Read the model definition and answer for the solid it produces. Units are mm, in the model's axes. A direction names the side the tool comes from. Give positions to 0.01 mm unless a question says otherwise; leave off trailing zeros. Order: outer loops, then holes, each group sorted by start corner. A loop starts at its lowest first (then second) coordinate and runs counter-clockwise, first axis right, second up.
Item 1: Find the intervals of material crossed by line 1 along Z through (x, y) = (12.7, 0) (3 decimals); line 2 along X through (y, z) = (-1.5, -346) (3 decimals); line 3 along Z through (x, y) = (231.5, 0) (3 decimals), in increasing order.
Item 2: A cutting plane is placed at B-B (x = 61.5). Write down the section's boundary in (y, z) (3 decimals).
Item 3: Given pin 1 Ø7.5 at (y, z) = (0, -447.675) entering from +X; pin 2 Ø1.5 at (x, y) = (140.5, 7) entering from -Z, each flat-ended and moving along its own axis, determine where each tip first touches the part or whether it passes through.
Item 4: The mould has two halves that part along X. Classify faces 1 (the face through (244.094, 0, -232)), 2 (the face through (225, 0, -457.2)), 3 (the face through (9.034, 0.133, -11.045)): +X half, -X half, draft (parallel to the pull), parting line (faces both ways), or undercut.
Item 5: A cutting plane is placed at C-C (y = 0). State how many separate pieces and enclosed holes the cut face has, plus the area to 3 significant figures.
Item 6: A cutting plane is placed at D-D (z = -101.6). Write down the section's boundary in (x, y) (3 decimals), plus the area to 3 significant figures.
Item 7: Which of the six approach directions +Z, -Z, +X, -X, +Y, -Y give full straight-line access (tool end or side, diameter ignored) to faces 4 (the face through (224.97, 1.377, -453.874)), 5 (the face through (202.556, 0.133, -212.278)), 6 (the face through (38.1, 0, -363))?
Item 8: A cutting plane is placed at A-A (z = -349). Write down the section's boundary in (x, y) (3 decimals).
from build123d import *

# Parameters (mm, degrees)
F0_W     = 168.275
F0_H     = 177.8
F1_DEPTH = 9.525
F3_D     = 12.7
F5_D     = 12.7
F7_D     = 7.9375
F8_R     = 12.7


# Not quite as in the source:
# - a length typed as a fraction of an inch, garbled in the dataset ("3 / 203.2 mm" for 3/8 in), is restored


with BuildPart() as f1:
    # F0 (on Front) → F1 (new body, symmetric)
    with BuildSketch(Plane.XZ):
        Polygon((244.094, 0), (0, 0), (0, -457.2), (38.1, -457.2), (38.1, -254), (206.375, -254), (206.375, -457.2), (244.094, -457.2), align=None)
        with Locations((122.2375, -127)):
            Rectangle(F0_W, F0_H, mode=Mode.SUBTRACT)
    extrude(amount=F1_DEPTH, both=True)

    # F3 (through all)
    with Locations(Plane.YZ.offset(244.094)):
        with Locations((0, -447.675)):
            Hole(F3_D / 2)

    # F5 (through all)
    with Locations(Plane.XZ.offset(9.525)):
        with Locations((12.7, -406.4), (12.7, -101.6)):
            Hole(F5_D / 2)

    # F7 (through all)
    with Locations(Plane.XZ.offset(9.525)):
        with Locations((12.7, -9.525), (12.7, -28.575), (231.394, -28.575), (231.394, -9.525)):
            Hole(F7_D / 2)

    # F8
    f8_edges = [f1.edges().sort_by_distance(p)[0] for p in [
        (38.1, 0, -38.1),
        (206.375, 0, -38.1),
        (206.375, 0, -215.9),
        (38.1, 0, -215.9),
        (206.375, 0, -254),
        (38.1, 0, -254),
    ]]
    fillet(f8_edges, radius=F8_R)


solid = f1.part
Response values:
1. line 1: z = -457.2 to -454.025, -441.325 to -412.75, -400.05 to -107.95, -95.25 to -32.544, -24.606 to -13.494, -5.556 to 0
1. line 2: x = 0 to 38.1, 206.375 to 244.094
1. line 3: z = -457.2 to -454.025, -441.325 to -32.542, -24.608 to -13.492, -5.558 to 0
2. outline: (-9.525, -254) - (9.525, -254) - (9.525, -215.9) - (-9.525, -215.9) - close; (-9.525, -38.1) - (9.525, -38.1) - (9.525, 0) - (-9.525, 0) - close
3. pin 1: passes through
3. pin 2: stops at z = -254
4. face 1: +X half
4. face 2: draft
4. face 3: undercut
5. separate pieces: 3
5. enclosed holes: 7
5. area: 46,300 mm2
6. outline: (0, -9.525) - (6.35, -9.525) - (6.35, 9.525) - (0, 9.525) - close; (19.05, -9.525) - (38.1, -9.525) - (38.1, 9.525) - (19.05, 9.525) - close; (206.375, -9.525) - (244.094, -9.525) - (244.094, 9.525) - (206.375, 9.525) - close
6. area: 1,200 mm2
7. face 4: +X, -X
7. face 5: +Y, -Y
7. face 6: -Z, +Y, -Y
8. outline: (0, -9.525) - (38.1, -9.525) - (38.1, 9.525) - (0, 9.525) - close; (206.375, -9.525) - (244.094, -9.525) - (244.094, 9.525) - (206.375, 9.525) - close
